Geometry: final body of the model. Coordinates: model frame, mm. A direction names the side the tool comes from. Coordinates: 2 decimals unless noted, no trailing zeros. Write each loop counter-clockwise with the first axis right and the second up, starting at its lowest first coordinate (ties: lowest second). Pieces come first, ordered by that corner, then holes. Notation, with made-up numbers: M 11.25,-36.5 L 46.25,-36.5 A11 ccw 46.25,-21.5 Z; hole C 10,58.5 d5. An arc over 180 degrees is marked long. Write item = value, one per line. Start each with the question number.
Item 1: Reachability of faces 4 (the flat face through (-21, 2, -9.125)), 5 (the conical face through (7.94, 0.62, -9.61)), 6 (the flat face through (-21, 2, 9.125)), 7 (the flat face through (21, 2, -9.125)), 8 (the flat face through (7.5, 2, 20)) from +Z, -Z, +X, -X, +Y, -Y: full face, straight path, thin tool, end or side. Return the list, or none.
Item 2: Section D-D on x = 14. Output: boundary loops of the cut face in (y, z) (3 decimals).
Item 3: First-contact query: pin 1 Ø0.6 at (y, z) = (1.5, -23.5) entering from -X; pin 2 Ø2 at (y, z) = (2, 22) entering from +X; pin 3 Ø1.6 at (x, y) = (-23, 2) entering from -Z (3 decimals). Flat tips, straight axial feed; report the tip coordinate or a pass-through.
Item 4: Ray query, L1, parallel to X at y = 1.4, z = 0 (3 decimals); L2, parallel to X at y = 1.15, z = -23; L3, parallel to X at y = 1.3, z = 2. Return the intervals inside material, ascending. Write a range as [from, to].
Item 5: Pull-direction query (X, two-part tool) for faces 1 (the flat face through (0, 2, 25.25)), 2 (the flat face through (21, 2, 9.125)), 3 (the conical face through (-6.36, 0.4, -29.08)); classes: +X half, -X half, draft (parallel to the pull), parting line (faces both ways), or undercut.
Item 6: Section A-A on z = -15. Output: boundary loops of the cut face in (x, y).
Item 7: Section C-C on x = 31. Output: boundary loops of the cut face in (y, z) (3 decimals), plus the area to 3 significant figures.
Item 8: Section B-B on z = 0. Output: boundary loops of the cut face in (x, y) (3 decimals).
from build123d import *

# Parameters (mm, degrees)
SKETCH1_R           = 4.125
SKETCH1_W           = 5
SKETCH1_H           = 50.5
BOSS_EXTRUDE1_DEPTH = 4
FILLET1_R           = 2.5
CHAMFER1_SIZE       = 1


with BuildPart() as part:
    # Sketch1 → Boss-Extrude1 (new body)
    with BuildSketch(Plane(origin=(0, 0, 0), x_dir=(1, 0, 0), z_dir=(0, 1, 0))):
        with BuildLine():
            Line((-32, 9.125), (-7.5, 9.125))
            Line((-7.5, 9.125), (-7.5, 30.25))
            Line((-7.5, 30.25), (7.5, 30.25))
            Line((7.5, 30.25), (7.5, 9.125))
            Line((7.5, 9.125), (32, 9.125))
            ThreePointArc((32, 9.125), (41.125, 0), (32, -9.125))
            Line((32, -9.125), (7.5, -9.125))
            Line((7.5, -9.125), (7.5, -30.25))
            Line((7.5, -30.25), (-7.5, -30.25))
            Line((-7.5, -30.25), (-7.5, -9.125))
            Line((-7.5, -9.125), (-32, -9.125))
            ThreePointArc((-32, -9.125), (-41.125, 0), (-32, 9.125))
        make_face()
        with Locations(Location((-32, 0, 0), (0, 0, 270))):
            Circle(SKETCH1_R, mode=Mode.SUBTRACT)
        with Locations(Location((32, 0, 0), (0, 0, 90))):
            Circle(SKETCH1_R, mode=Mode.SUBTRACT)
        Rectangle(SKETCH1_W, SKETCH1_H, mode=Mode.SUBTRACT)
    extrude(amount=BOSS_EXTRUDE1_DEPTH)

    # Fillet1
    fillet1_edges = [part.edges().sort_by_distance(p)[0] for p in [
        (-7.5, 2, -9.125),
        (-7.5, 2, -30.25),
        (7.5, 2, -30.25),
        (7.5, 2, -9.125),
        (7.5, 2, 9.125),
        (7.5, 2, 30.25),
        (-7.5, 2, 30.25),
        (-7.5, 2, 9.125),
    ]]
    fillet(fillet1_edges, radius=FILLET1_R)

    # Chamfer1
    chamfer1_edges = [part.edges().sort_by_distance(p)[0] for p in [
        (21, 0, -9.125),
        (41.125, 0, 0),
        (-21, 0, 9.125),
        (-41.125, 0, 0),
        (41.125, 4, 0),
        (21, 4, -9.125),
        (-41.125, 4, 0),
        (-7.5, 0, 19.6875),
        (-7.5, 4, 19.6875),
        (0, 0, 30.25),
        (0, 4, 30.25),
        (-21, 0, -9.125),
        (-7.5, 0, -19.6875),
        (0, 0, -30.25),
        (7.5, 0, -19.6875),
        (21, 0, 9.125),
        (7.5, 0, 19.6875),
        (-6.767766953, 0, -29.517766953),
        (6.767766953, 0, -29.517766953),
        (6.767766953, 0, 29.517766953),
        (-6.767766953, 0, 29.517766953),
        (7.5, 4, 19.6875),
        (21, 4, 9.125),
        (7.5, 4, -19.6875),
        (0, 4, -30.25),
        (-7.5, 4, -19.6875),
        (-21, 4, -9.125),
        (-6.767766953, 4, -29.517766953),
        (6.767766953, 4, -29.517766953),
        (6.767766953, 4, 29.517766953),
        (-6.767766953, 4, 29.517766953),
        (-8.232233047, 0, 9.857233047),
        (-8.232233047, 4, 9.857233047),
        (8.232233047, 0, 9.857233047),
        (8.232233047, 4, 9.857233047),
        (8.232233047, 0, -9.857233047),
        (8.232233047, 4, -9.857233047),
        (-8.232233047, 0, -9.857233047),
        (-8.232233047, 4, -9.857233047),
        (-21, 4, 9.125),
    ]]
    chamfer(chamfer1_edges, length=CHAMFER1_SIZE)


solid = part.part
Responses:
q1.face_4 = -Z, -X, +Y, -Y
q1.face_5 = -Z, +X, -Y
q1.face_6 = +Z, -X, +Y, -Y
q1.face_7 = -Z, +X, +Y, -Y
q1.face_8 = +Z, +X, +Y, -Y
q2.outline = M 0,-8.125 L 1,-9.125 L 3,-9.125 L 4,-8.125 L 4,8.125 L 3,9.125 L 1,9.125 L 0,8.125 Z
q3.pin_1 = -7.5
q3.pin_2 = 7.5
q3.pin_3 = -9.125
q4.L1 = [-41.125, -36.125], [-27.875, -2.5], [2.5, 27.875], [36.125, 41.125]
q4.L2 = [-7.5, -2.5], [2.5, 7.5]
q4.L3 = [-40.9, -35.61], [-28.39, -2.5], [2.5, 28.39], [35.61, 40.9]
q5.face_1 = undercut
q5.face_2 = draft
q5.face_3 = -X half
q6.outline = M -7.5,1 L -6.5,0 L -2.5,0 L -2.5,4 L -6.5,4 L -7.5,3 Z; M 2.5,0 L 6.5,0 L 7.5,1 L 7.5,3 L 6.5,4 L 2.5,4 Z
q7.outline = M 0,-8.125 L 1,-9.125 L 3,-9.125 L 4,-8.125 L 4,-4.002 L 0,-4.002 Z; M 0,4.002 L 4,4.002 L 4,8.125 L 3,9.125 L 1,9.125 L 0,8.125 Z
q7.area = 39.0 mm²
q8.outline = M -41.125,1 L -40.125,0 L -36.125,0 L -36.125,4 L -40.125,4 L -41.125,3 Z; M -27.875,0 L -2.5,0 L -2.5,4 L -27.875,4 Z; M 2.5,0 L 27.875,0 L 27.875,4 L 2.5,4 Z; M 36.125,0 L 40.125,0 L 41.125,1 L 41.125,3 L 40.125,4 L 36.125,4 Z
